Could you check a few things on this model? Use its own coordinates, in mm. A direction names the side the tool comes from. Give positions to 0.01 mm unless a question says otherwise; leave off trailing zeros. Loops run counter-clockwise (first coordinate to the right, second up) from the corner with the lowest first, then second, coordinate; pieces in that order, holes last. Notation, with made-up numbers: M 19,26.5 L 49,26.5 A23 ccw 49,35.5 Z; hole C 32.25,56 d11. An arc over 180 degrees is marked long. Answer in a Markdown table with one row per item. Add a question column.
1. Which directions (+Z, -Z, +X, -X, +Y, -Y) give clear straight access to the entire face, cutting with the end or side of a thin tool? Please do faces 5 (the flat face through (-5, 18, 0)), 6 (the flat face through (2.5, 0, -2.5)), 7 (the cylindrical face through (0.173, 14.997, 7.872)), 8 (the cylindrical face through (-0.061, 16.571, -2.793)), 9 (the flat face through (5, 18, 0)).
2. If we section it at A-A on y = 3.5: List the corners of the cut face in (x, z) for me, then the cut area to 3 significant figures.
3. If we section it at C-C on y = 18.5: List the corners of the cut face in (x, z) for me.
4. If we section it at B-B on z = 4.5: Count the separate pieces of the cut face and the enclosed holes in it, then the cut area to 3 significant figures.
5. If we section it at D-D on y = 21.25: List the corners of the cut face in (x, z) for me, then the cut area to 3 significant figures.
6. I need wall thicknesses on line 1 along Y through (x, z) = (-4.5, -9.75); line 2 along Z through (x, y) = (5.75, 0.25); line 3 along Z through (x, y) = (-0.25, 10.25). Which ranges of each line are inside material? Lowest first, please. Write a range as from..to.
7. I'm going to push flat-ended pins straight in: pin 1 Ø1 at (x, z) = (4.5, 4.5) entering from -Y; pin 2 Ø1.5 at (y, z) = (9.5, -6) entering from -X; pin 3 Ø4 at (x, y) = (4.5, 5.5) entering from +Z. Where does each tip first touch, or does it pass through?
8. Thinking about a two-plate mould opening in Y: for faces 1 (the flat face through (1, 13.462, -1)), 2 (the flat face through (-3, 12.446, 2)), 3 (the flat face through (0, 20.472, 2)), 4 (the cylindrical face through (-0.061, 18.146, -2.793)), which applies, released by +Y, released by -Y, zero draft, split by the parting line, or undercut?
```python
from build123d import *

# Parameters (mm, degrees)
SKETCH1_W           = 1.016
SKETCH1_H           = 10.922
SKETCH1_W_2         = 3.048
SKETCH1_H_2         = 1.524
FILLET1_R           = 1.27
BOSS_EXTRUDE1_DEPTH = 0.762
LPATTERN1_COUNT     = 4
LPATTERN1_PITCH     = 1.5748


with BuildPart() as part:
    # Sketch1 → Revolve1 (revolve)
    with BuildSketch(Plane.XY, mode=Mode.PRIVATE) as revolve1_sk:
        Polygon((-3.302, 13.462), (0, 13.462), (0, 0), (-11.938, 0), (-11.938, 12.446), (-3.302, 12.446), align=None)
        with Locations((-0.508, 18.923)):
            Rectangle(SKETCH1_W, SKETCH1_H)
        with Locations((-1.524, -0.762)):
            Rectangle(SKETCH1_W_2, SKETCH1_H_2)
    revolve(revolve1_sk.sketch.rotate(Axis((0, 0, 0), (0, -1, 0)), 270), axis=Axis((0, 0, 0), (0, -1, 0)))

    # Fillet1
    fillet1_edges = [part.edges().sort_by_distance(p)[0] for p in [
        (0, -1.524, -3.048),
        (0, 12.446, -11.938),
    ]]
    fillet(fillet1_edges, radius=FILLET1_R)

    # Sketch2 → Boss-Extrude1 (add, symmetric)
    with BuildSketch(Plane(origin=(0, 14.986, 0), x_dir=(1, 0, 0), z_dir=(0, 1, 0))):
        with BuildLine():
            Line((-7.874, 0), (-2.794, 0))
            ThreePointArc((-2.794, 0), (0, 2.794), (2.794, 0))
            Line((2.794, 0), (7.874, 0))
            ThreePointArc((7.874, 0), (0, -7.874), (-7.874, 0))
        make_face()
    boss_extrude1 = extrude(amount=BOSS_EXTRUDE1_DEPTH, both=True)

    # LPattern1: Boss-Extrude1 ×4
    with Locations(*[(0, i * LPATTERN1_PITCH, 0) for i in range(1, LPATTERN1_COUNT)]):
        add(boss_extrude1)


solid = part.part
```
Results:
| question | item | result |
|---|---|---|
| 1 | face 5 | -Z, -X, +Y |
| 1 | face 6 | -Y |
| 1 | face 7 | +Z, +Y |
| 1 | face 8 | -Z, +Y |
| 1 | face 9 | -Z, +X, +Y |
| 2 | outline | C 0,0 d23.88 |
| 2 | area | 448 mm2 |
| 3 | outline | M -7.87,0 L -2.79,0 A2.79 ccw 2.79,0 L 7.87,0 A7.87 ccw Z |
| 4 | separate pieces | 5 |
| 4 | enclosed holes | 0 |
| 4 | area | 353 mm2 |
| 5 | outline | C 0,0 d2.03 |
| 5 | area | 3.24 mm2 |
| 6 | line 1 | 0..12.44 |
| 6 | line 2 | -10.46..10.46 |
| 6 | line 3 | -11.94..11.94 |
| 7 | pin 1 | y = 0 |
| 7 | pin 2 | x = -10.72 |
| 7 | pin 3 | z = 11.67 |
| 8 | face 1 | undercut |
| 8 | face 2 | undercut |
| 8 | face 3 | released by +Y |
| 8 | face 4 | zero draft |
